Input: dimensioned drawing with shaded views. Units: mm. Origin: part minimum x, y, z. A direction names the side the tool comes from. Round coordinates to 2 decimals unless told otherwise and drop trailing zeros. Loops run counter-clockwise (first coordinate to the right, second up) from the corner with the lowest first, then second, coordinate; pieces in that order, holes last.
1) First-contact query: pin 1 (1 mm diameter, centred on x = 8.5, z = 13, fed in from -Y); pin 2 (2 mm diameter, centred on x = 30.5, y = 12.5, fed in from -Z). Flat tips, straight axial feed; report the tip coordinate or a pass-through.
2) Section A-A, the plane z = 16. Return loops of the section in (x, y).
3) Section B-B, the plane x = 40. Return loops of the section in (y, z), and give its area (3 significant figures).
4) Access query for the marked faces 1 and 2. Directions: +Z, -Z, +X, -X, +Y, -Y. A direction counts if a zero-diameter tool reaches every point of the face in a straight line with its end or side. Return the directions, or none.
5) Ray query, line 1 along Z through (x, y) = (28, 41.5); line 2 along Y through (x, z) = (14.5, 8). Return the intervals inside material, ascending.
6) Section C-C, the plane y = 24. Return loops of the section in (x, z).
7) Section D-D, the plane x = 50.5. Return loops of the section in (y, z), and give its area (3 significant figures).
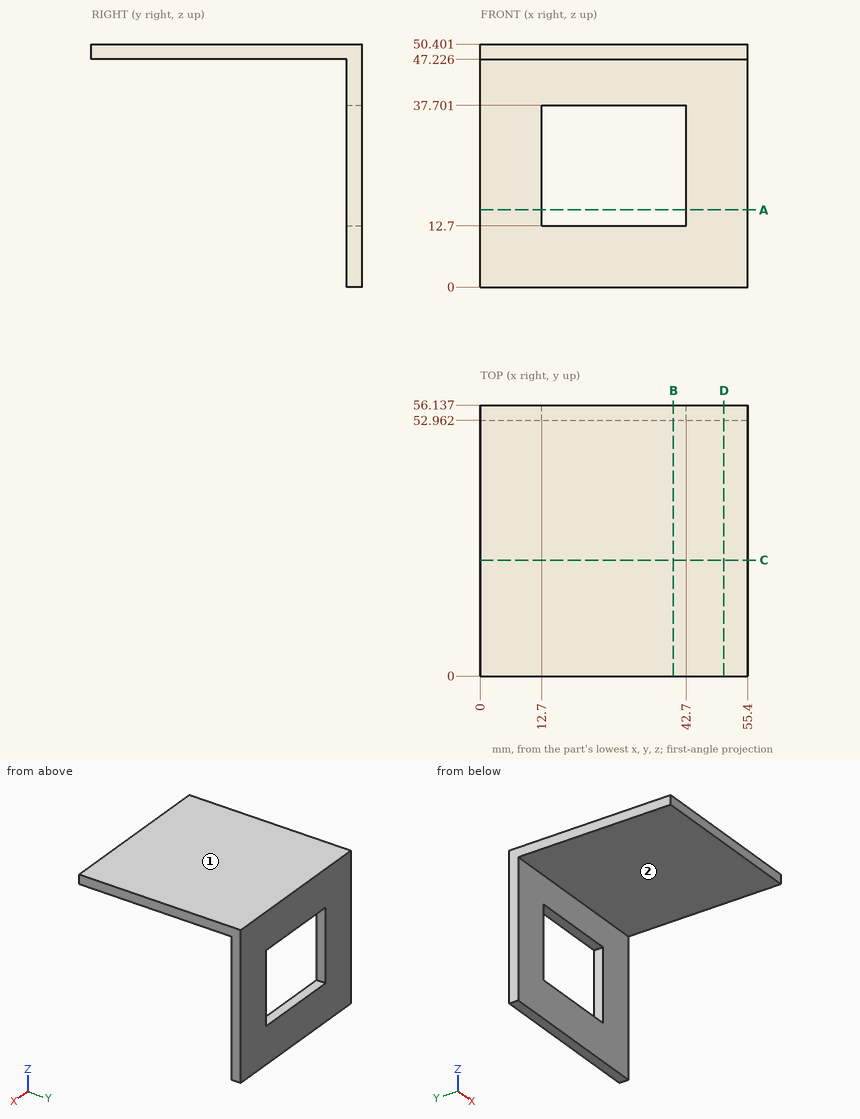
Final values:
1. pin 1: stops at y = 52.96
1. pin 2: stops at z = 47.23
2. outline: (0, 52.96) - (12.7, 52.96) - (12.7, 56.14) - (0, 56.14) - close; (42.7, 52.96) - (55.4, 52.96) - (55.4, 56.14) - (42.7, 56.14) - close
3. outline: (0, 47.23) - (52.96, 47.23) - (52.96, 37.7) - (56.14, 37.7) - (56.14, 50.4) - (0, 50.4) - close; (52.96, 0) - (56.14, 0) - (56.14, 12.7) - (52.96, 12.7) - close
3. area: 249 mm2
4. face 1: +Z, +X, -X, +Y, -Y
4. face 2: -Z, +X, -X, -Y
5. line 1: z = 47.23 to 50.4
5. line 2: y = 52.96 to 56.14
6. outline: (0, 47.23) - (55.4, 47.23) - (55.4, 50.4) - (0, 50.4) - close
7. outline: (0, 47.23) - (52.96, 47.23) - (52.96, 0) - (56.14, 0) - (56.14, 50.4) - (0, 50.4) - close
7. area: 328 mm2
